Read the model definition and answer for the solid it produces. Units are mm, in the model's axes. A direction names the side the tool comes from. Give positions to 0.01 mm unless a question says otherwise; leave off trailing zeros. Write each loop counter-clockwise with the first axis right and the second up, starting at its lowest first coordinate (ties: lowest second). Pieces come first, ordered by that corner, then holes. Notation, with made-up numbers: (28, 67.5) -> (37, 67.5) arc R19 ccw to (37, 99.5) -> close; hole circle Ø2 at (-20.75, 30.5). An arc over 180 degrees is marked (long way). Put each result on its own line as item: value. Start each with the question number.
Autodesk Inventor part; units mm, degrees
ref_plane "YZ Plane" through (0, 0, 0) normal (1, 0, 0) x (0, 1, 0)
ref_plane "XZ Plane" through (0, 0, 0) normal (0, 1, 0) x (-1, 0, 0)
ref_plane "XY Plane" through (0, 0, 0) normal (0, 0, 1) x (1, 0, 0)
sketch "Szkic1" plane through (0, 0, 0) normal (0, 1, 0) x (-1, 0, 0)
  circle A0 centre (0, 0) radius 1.5
  circle A1 centre (0, 0) radius 5
  line L0 (5, 0) -> (-5, 0)
  line L1 (-5, 0) -> (-5, -6)
  line L2 (-5, -6) -> (5, -6)
  line L3 (5, -6) -> (5, 0)
  dimension "d1" = 10
  dimension "d0" = 3
  dimension "d2" = 6
extrude "Wyciągnięcie proste1" add sketch "Szkic1" along normal blind 5
sketch "Szkic2" plane through (5, 0, -6) normal (0, 0, -1) x (-1, 0, 0)
  line L0 (0, 0) -> (10, 0)
  line L1 (10, 0) -> (10, 5)
  line L2 (0, 5) -> (10, 5)
  line L3 (0, 0) -> (0, 5)
  line L4 (0, 5) -> (10, 5)
  line L5 (10, 5) -> (10, -5)
  line L6 (10, -5) -> (0, -5)
  line L7 (0, -5) -> (0, 5)
  point P0 (5, 0)
  dimension "d5" = 5
extrude "Wyciągnięcie proste2" add sketch "Szkic2" along normal blind 3
sketch "Szkic3" plane through (0, 5, 0) normal (0, 1, 0) x (1, 0, 0)
  point P0 (0, 0)
  point P1 (0, 0)
hole "Otwór1" at (0, 5, 0) direction (0, -1, 0) diameter 3.5 end through all counterbore diameter 6 counterbore depth 2
properties part number "podpora_lewa"
1) A cutting plane is placed at D-D on x = -1.25. Give the vertices of the cut face in (y, z).
2) A cutting plane is placed at A-A on x = 0. Give the vertices of the cut face in (y, z).
3) Each of these flat-tipped pins is pushed along its axis until it touches: pin 1 Ø5.5 at (x, y) = (0.5, -3.5) entering from +Z; pin 2 Ø5 at (x, y) = (-2, -2) entering from +Z. Where does it stop, or does it pass through?
4) A cutting plane is placed at B-B on z = -0.25. Give the vertices of the cut face in (x, y).
5) For a pull along Z with two mould halves and no side action, classify faces 1 (the face through (0.67, 1.479, 1.617)), 2 (the face through (0.1, 5, -3.5)), 3 (the face through (0, 2, 5)) as pulls with the +Z half, pulls with the -Z half, needs draft (parallel to the pull), parting line crosses it, or undercut.
6) Straight lines are drawn through the part: line 1 (Z direction, x = 0, y = 3.5); line 2 (Z direction, x = 0, y = 0.7); line 3 (X direction, y = 4.2, z = 0). For each, find the intervals that lie inside material, in ascending order. Write a range as [from, to].
7) A cutting plane is placed at C-C on y = 1. Give the vertices of the cut face in (x, z).
8) For faces 4 (the face through (-5, 1, -6)), 5 (the face through (2, 3, 0)), 6 (the face through (-1, 0, -2)), determine the directions among +Z, -Z, +X, -X, +Y, -Y from which every point of the face is accessible in a straight line to the end or side of a thin tool.
Results found:
1. outline: (-5, -9) -> (5, -9) -> (5, -2.73) -> (3, -2.73) -> (3, -1.22) -> (0, -1.22) -> (0, -6) -> (-5, -6) -> close; (0, 1.22) -> (3, 1.22) -> (3, 2.73) -> (5, 2.73) -> (5, 4.84) -> (0, 4.84) -> close
2. outline: (-5, -9) -> (5, -9) -> (5, -3) -> (3, -3) -> (3, -1.75) -> (0, -1.75) -> (0, -6) -> (-5, -6) -> close; (0, 1.75) -> (3, 1.75) -> (3, 3) -> (5, 3) -> (5, 5) -> (0, 5) -> close
3. pin 1: stops at z = -6
3. pin 2: stops at z = 4.97
4. outline: (-5, 0) -> (-1.73, 0) -> (-1.73, 3) -> (-2.99, 3) -> (-2.99, 5) -> (-5, 5) -> close; (1.73, 0) -> (5, 0) -> (5, 5) -> (2.99, 5) -> (2.99, 3) -> (1.73, 3) -> close
5. face 1: undercut
5. face 2: needs draft
5. face 3: pulls with the +Z half
6. line 1: z = [-9, -3], [3, 5]
6. line 2: z = [-9, -1.75], [1.75, 5]
6. line 3: x = [-5, -3], [3, 5]
7. outline: (-5, -9) -> (5, -9) -> (5, 0) arc R5 ccw to (-5, 0) -> close; hole circle Ø3.5 at (0, 0)
8. face 4: +Z, -Z, -X, +Y, -Y
8. face 5: +Y
8. face 6: +Z, +X, -X, -Y
